Design review of the part built by this model. Coordinates are the model's own, in mm. A direction names the side the tool comes from. Coordinates: 2 decimals unless noted, no trailing zeros. Order: outer loops, then holes, each group sorted by start corner. A loop starts at its lowest first (then second) coordinate and runs counter-clockwise, first axis right, second up. Notation, with made-up numbers: (-27.5, 79.5) - (-12.5, 79.5) arc R17 ccw to (-12.5, 84.5) - close; hole circle Ø7 at (78.5, 58.5). An arc over 180 degrees is marked (long way). Write item = value, one per line. Start each with the question number.
```python
from build123d import *

# Parameters (mm, degrees)
EXTRUDE_1_DEPTH = 8
FILLET_1_R      = 0.2


with BuildPart() as part:
    # Эскиз1 → Бобышка-Вытянуть1 (new body, symmetric)
    with BuildSketch(Plane.XY):
        Polygon((4, 0), (-4, 0), (-4, -1.8), (-8, -1.8), (-8, -3.6), (-4, -6), (4, -6), (8, -3.6), (8, -1.8), (4, -1.8), align=None)
    extrude(amount=EXTRUDE_1_DEPTH, both=True)

    # Эскиз4 → Отверстие обработанное метчиком M62 (revolve, cut)
    with BuildSketch(Plane(origin=(0, 0, 0), x_dir=(0, 0, 1), z_dir=(1, 0, 0))):
        Polygon((0, 0), (0, 6), (3.025, 6), (2.5, 5.475), (2.5, 0.525), (3.025, 0), align=None)
    revolve(axis=Axis((0, 6.35, 0), (0, -1, 0)), mode=Mode.SUBTRACT)

    # Скругление1
    fillet_1_edges = [part.edges().sort_by_distance(p)[0] for p in [
        (-4, 0, 0),
        (4, 0, 0),
        (4, -1.8, 0),
        (8, -1.8, 0),
        (4, -6, 0),
        (-4, -6, 0),
        (-8, -1.8, 0),
        (-4, -1.8, 0),
    ]]
    fillet(fillet_1_edges, radius=FILLET_1_R)


solid = part.part
```
Item 1: For line 1 (X direction, y = -2.85, z = 0); line 2 (X direction, y = -1.6, z = 0), list the stretches that pass through material, from the lowest coordinate up.
Item 2: Add section D-D on z = 3.25. Give the boundary of the cut face in (x, y), plus the area to 3 significant figures.
Item 3: For faces 1 (the flat face through (-4, -1, 0)), 2 (the flat face through (3, 0, 2)), 3 (the flat face through (6, -1.8, 0)), list the 3-axis set-ups (+Z, -Z, +X, -X, +Y, -Y) from which the entire face can be reached by the end or side of a thin tool; tool diameter is ignored.
Item 4: Add section C-C on y = -4.05. Give the boundary of the cut face in (x, z).
Item 5: Add section A-A on x = 0. Give the boundary of the cut face in (y, z) (3 decimals), plus the area to 3 significant figures.
Item 6: Mouldability with a two-part tool opening along X and no side actions: class faces 4 (the cylindrical face through (2.44, -2.97, -0.54)), 5 (the flat face through (-6, -1.8, 0)), 6 (the flat face through (4, -1, 0)) as +X half, -X half, draft (parallel to the pull), parting line (faces both ways), or undercut.
Item 7: For P1, Ø4, axis at x = 6.5, z = 0, coming from the +Y side; P2, Ø2, axis at x = 6, z = 1.5, coming from the -Y side; P3, Ø0.7, axis at y = -1, z = 3.5, coming from the +X side, all flat-tipped, find the tip position at first contact; note any pin that passes through.
Worked out:
q1.line_1 = -8 to -2.5, 2.5 to 8
q1.line_2 = -4 to -2.5, 2.5 to 4
q2.outline = (-8, -3.6) - (-4.05, -5.97) arc R0.2 ccw to (-3.94, -6) - (3.94, -6) arc R0.2 ccw to (4.05, -5.97) - (8, -3.6) - (8, -2) arc R0.2 ccw to (7.8, -1.8) - (4.2, -1.8) arc R0.2 cw to (4, -1.6) - (4, -0.2) arc R0.2 ccw to (3.8, 0) - (-3.8, 0) arc R0.2 ccw to (-4, -0.2) - (-4, -1.6) arc R0.2 cw to (-4.2, -1.8) - (-7.8, -1.8) arc R0.2 ccw to (-8, -2) - close
q2.area = 72.0 mm2
q3.face_1 = +Z, -Z, -X, +Y
q3.face_2 = +Z, -Z, +X, -X, +Y
q3.face_3 = +Z, -Z, +X, +Y
q4.outline = (-7.25, -8) - (7.25, -8) - (7.25, 8) - (-7.25, 8) - close; hole circle Ø5 at (0, 0)
q5.outline = (-6, -8) - (0, -8) - (0, -3.025) - (-0.525, -2.5) - (-5.475, -2.5) - (-6, -3.025) - close; (-6, 3.025) - (-5.475, 2.5) - (-0.525, 2.5) - (0, 3.025) - (0, 8) - (-6, 8) - close
q5.area = 65.4 mm2
q6.face_4 = undercut
q6.face_5 = draft
q6.face_6 = +X half
q7.P1 = -1.8
q7.P2 = -5.4
q7.P3 = 4
